Input: part model. Units: mm. Frame: model coordinates. A direction names the side the tool comes from. Give positions to 0.01 mm unless a question says otherwise; leave off trailing zeros. Order: outer loops, then holes, each group sorted by start corner. A loop starts at its lowest first (then second) coordinate and runs counter-clockwise, first axis right, second up. Notation, with made-up numbers: (44, 73) - (73, 73) arc R21 cw to (73, 90) - close; hole circle Ø3 at (29.25, -0.75). An arc over 180 degrees is marked (long way). Use a Markdown table: item, result.
from build123d import *

# Parameters (mm, degrees)
SKETCH1_W           = 22.9
SKETCH1_H           = 12.4968
BOSS_EXTRUDE1_DEPTH = 5.08
SKETCH2_W           = 22.9
SKETCH2_H           = 2.286
BOSS_EXTRUDE2_DEPTH = 1.016
SKETCH3_W           = 1.016
SKETCH3_H           = 1.016
CUT_EXTRUDE1_DEPTH  = 27.577930887
SKETCH4_W           = 20.2184
SKETCH4_H           = 2.4638
BOSS_EXTRUDE3_DEPTH = 6.8072
SKETCH5_W           = 7.62
SKETCH5_H           = 8.128
BOSS_EXTRUDE4_DEPTH = 2.8702
BOSS_EXTRUDE6_DEPTH = 1.778


with BuildPart() as part:
    # Sketch1 → Boss-Extrude1 (new body)
    with BuildSketch(Plane(origin=(0, 0, 0), x_dir=(1, 0, 0), z_dir=(0, 1, 0))):
        with Locations((11.45, 6.2484)):
            Rectangle(SKETCH1_W, SKETCH1_H)
    extrude(amount=BOSS_EXTRUDE1_DEPTH)

    # Sketch2 → Boss-Extrude2 (add)
    with BuildSketch(Plane.XY):
        with Locations((11.45, 2.449418531)):
            Rectangle(SKETCH2_W, SKETCH2_H)
    extrude(amount=BOSS_EXTRUDE2_DEPTH)

    # Sketch3 → Cut-Extrude1 (cut, through all)
    with BuildSketch(Plane(origin=(0, 5.08, 0), x_dir=(1, 0, 0), z_dir=(0, 1, 0))):
        with Locations((2.56, -0.508)):
            Rectangle(SKETCH3_W, SKETCH3_H)
        with Locations((5.1, -0.508)):
            Rectangle(SKETCH3_W, SKETCH3_H)
        with Locations((7.64, -0.508)):
            Rectangle(SKETCH3_W, SKETCH3_H)
        with Locations((10.18, -0.508)):
            Rectangle(SKETCH3_W, SKETCH3_H)
        with Locations((12.72, -0.508)):
            Rectangle(SKETCH3_W, SKETCH3_H)
        with Locations((15.26, -0.508)):
            Rectangle(SKETCH3_W, SKETCH3_H)
        with Locations((17.8, -0.508)):
            Rectangle(SKETCH3_W, SKETCH3_H)
        with Locations((20.34, -0.508)):
            Rectangle(SKETCH3_W, SKETCH3_H)
    extrude(amount=-CUT_EXTRUDE1_DEPTH, mode=Mode.SUBTRACT)

    # Sketch4 → Boss-Extrude3 (add)
    with BuildSketch(Plane(origin=(0, 0, -12.4968), x_dir=(-1, 0, 0), z_dir=(0, 0, -1))):
        with Locations((-11.45, 2.54)):
            Rectangle(SKETCH4_W, SKETCH4_H)
    extrude(amount=BOSS_EXTRUDE3_DEPTH)

    # Sketch5 → Boss-Extrude4 (add)
    with BuildSketch(Plane(origin=(0, 3.7719, 0), x_dir=(1, 0, 0), z_dir=(0, 1, 0))):
        with Locations((11.45, 12.6746)):
            Rectangle(SKETCH5_W, SKETCH5_H)
    extrude(amount=BOSS_EXTRUDE4_DEPTH)

    # Sketch6 → Boss-Extrude6 (add)
    # profile 1 of 4: a face of its own
    with BuildSketch(Plane(origin=(0, 3.7719, 0), x_dir=(1, 0, 0), z_dir=(0, 1, 0))):
        with BuildLine():
            add(Edge.make_bspline(
                [(12.764837987, 19.304), (12.764837987, 19.513213272), (12.713813556, 19.940397022), (12.430473546, 20.689983513), (11.84369856, 21.434451274), (10.99868157, 22.128872758), (10.114149769, 22.755114216), (9.290977221, 23.379772734), (8.634141686, 24.039902479), (8.28695824, 24.637071385), (8.136269303, 25.170420647), (8.107573693, 25.497240703), (8.107573693, 25.654)],
                knots=[0, 0, 0, 0, 0.0625, 0.125, 0.25, 0.375, 0.5, 0.625, 0.75, 0.875, 0.9375, 1, 1, 1, 1], degree=3))
            Line((8.107573693, 25.654), (8.107573693, 28.829))
            Line((8.107573693, 28.829), (5.821803018, 28.829))
            Line((5.821803018, 28.829), (5.821803018, 25.672693301))
            add(Edge.make_bspline(
                [(1.842837987, 19.304), (1.842837987, 22.316040756), (5.821803018, 22.055802608), (5.821803018, 25.672693301)],
                knots=[0, 0, 0, 0, 1, 1, 1, 1], degree=3))
            Line((1.842837987, 19.304), (2.604837987, 19.304))
            add(Edge.make_bspline(
                [(2.604837987, 19.304), (2.604837987, 19.436184229), (2.628829628, 19.717403115), (2.748821923, 20.134038551), (3.017012948, 20.581214899), (3.561863063, 21.101594101), (4.28319589, 21.642805815), (5.083141911, 22.269605528), (5.750459382, 22.975833182), (6.10677757, 23.58043805), (6.230115453, 23.859247989), (6.250774433, 23.908581669)],
                knots=[0, 0, 0, 0, 0.0625, 0.125, 0.25, 0.375, 0.5, 0.625, 0.75, 0.824094442, 0.839719442, 0.839719442, 0.839719442, 0.839719442], degree=3))
            add(Edge.make_bspline(
                [(6.250774433, 23.908581669), (6.271433413, 23.95791535), (6.316227133, 24.071064885), (6.41779978, 24.365489751), (6.480855857, 24.623522586), (6.514810758, 24.824299603)],
                knots=[0.839719442, 0.839719442, 0.839719442, 0.839719442, 0.855344442, 0.875, 0.928476516, 0.928476516, 0.928476516, 0.928476516], degree=3))
            add(Edge.make_bspline(
                [(6.300749052, 23.880300217), (6.391194329, 24.164866019), (6.464932294, 24.476628676), (6.514810758, 24.824299603)],
                knots=[0.790040378, 0.790040378, 0.790040378, 0.790040378, 0.909912617, 0.909912617, 0.909912617, 0.909912617], degree=3))
            add(Edge.make_bspline(
                [(4.382837987, 19.304), (4.382837987, 21.310686016), (5.704652562, 22.004816166), (6.300749052, 23.880300217)],
                knots=[0, 0, 0, 0, 0.790040378, 0.790040378, 0.790040378, 0.790040378], degree=3))
            Line((4.382837987, 19.304), (5.144837987, 19.304))
            add(Edge.make_bspline(
                [(5.144837987, 19.304), (5.144837987, 19.427793819), (5.158559892, 19.685949652), (5.231289869, 20.113666624), (5.394061657, 20.587818607), (5.695490865, 21.140525626), (6.088197228, 21.743923542), (6.524741922, 22.447977177), (6.93514926, 23.302596179), (7.174536626, 24.122966736), (7.269542471, 24.705079276), (7.293215165, 24.899470513), (7.299029307, 24.951977964)],
                knots=[0, 0, 0, 0, 0.0625, 0.125, 0.25, 0.375, 0.5, 0.625, 0.75, 0.875, 0.918103341, 0.933728341, 0.933728341, 0.933728341, 0.933728341], degree=3))
            add(Edge.make_bspline(
                [(7.299029307, 24.951977964), (7.304843448, 25.004485416), (7.327450173, 25.230534496), (7.341165481, 25.474360975), (7.345573693, 25.654)],
                knots=[0.933728341, 0.933728341, 0.933728341, 0.933728341, 0.949353341, 1, 1, 1, 1], degree=3))
            add(Edge.make_bspline(
                [(7.417250324, 24.951977964), (7.370695979, 25.171529954), (7.345573693, 25.404885005), (7.345573693, 25.654)],
                knots=[0.926554678, 0.926554678, 0.926554678, 0.926554678, 1, 1, 1, 1], degree=3))
            add(Edge.make_bspline(
                [(12.002837987, 19.304), (12.002837987, 21.609223862), (8.004559962, 22.182204254), (7.417250324, 24.951977964)],
                knots=[0, 0, 0, 0, 0.926554678, 0.926554678, 0.926554678, 0.926554678], degree=3))
            Line((12.002837987, 19.304), (12.764837987, 19.304))
        make_face()
        with BuildLine():
            add(Edge.make_bspline(
                [(6.514810758, 24.824299603), (6.520540217, 24.858178177), (6.563211161, 25.129441995), (6.583803018, 25.423501077), (6.583803018, 25.672693301)],
                knots=[0.928476516, 0.928476516, 0.928476516, 0.928476516, 0.9375, 1, 1, 1, 1], degree=3))
            add(Edge.make_bspline(
                [(6.514810758, 24.824299603), (6.552295837, 25.08558415), (6.576305195, 25.367149502), (6.583803018, 25.672693301)],
                knots=[0.909912617, 0.909912617, 0.909912617, 0.909912617, 1, 1, 1, 1], degree=3))
        make_face(mode=Mode.SUBTRACT)
    # profile 2 of 4: a face of its own
    with BuildSketch(Plane(origin=(0, 3.7719, 0), x_dir=(1, 0, 0), z_dir=(0, 1, 0))):
        with BuildLine():
            Line((7.299029307, 24.951977964), (7.417250324, 24.951977964))
            add(Edge.make_bspline(
                [(7.417250324, 24.951977964), (7.370695979, 25.171529954), (7.345573693, 25.404885005), (7.345573693, 25.654)],
                knots=[0.926554678, 0.926554678, 0.926554678, 0.926554678, 1, 1, 1, 1], degree=3))
            add(Edge.make_bspline(
                [(7.299029307, 24.951977964), (7.304843448, 25.004485416), (7.327450173, 25.230534496), (7.341165481, 25.474360975), (7.345573693, 25.654)],
                knots=[0.933728341, 0.933728341, 0.933728341, 0.933728341, 0.949353341, 1, 1, 1, 1], degree=3))
        make_face()
    # profile 3 of 4: a face of its own
    with BuildSketch(Plane(origin=(0, 3.7719, 0), x_dir=(1, 0, 0), z_dir=(0, 1, 0))):
        with BuildLine():
            Line((6.250774433, 23.908581669), (6.300749052, 23.880300217))
            add(Edge.make_bspline(
                [(6.300749052, 23.880300217), (6.391194329, 24.164866019), (6.464932294, 24.476628676), (6.514810758, 24.824299603)],
                knots=[0.790040378, 0.790040378, 0.790040378, 0.790040378, 0.909912617, 0.909912617, 0.909912617, 0.909912617], degree=3))
            add(Edge.make_bspline(
                [(6.250774433, 23.908581669), (6.271433413, 23.95791535), (6.316227133, 24.071064885), (6.41779978, 24.365489751), (6.480855857, 24.623522586), (6.514810758, 24.824299603)],
                knots=[0.839719442, 0.839719442, 0.839719442, 0.839719442, 0.855344442, 0.875, 0.928476516, 0.928476516, 0.928476516, 0.928476516], degree=3))
        make_face()
    # profile 4 of 4: a face of its own
    with BuildSketch(Plane(origin=(0, 3.7719, 0), x_dir=(1, 0, 0), z_dir=(0, 1, 0))):
        with BuildLine():
            add(Edge.make_bspline(
                [(6.514810758, 24.824299603), (6.552295837, 25.08558415), (6.576305195, 25.367149502), (6.583803018, 25.672693301)],
                knots=[0.909912617, 0.909912617, 0.909912617, 0.909912617, 1, 1, 1, 1], degree=3))
            add(Edge.make_bspline(
                [(6.514810758, 24.824299603), (6.520540217, 24.858178177), (6.563211161, 25.129441995), (6.583803018, 25.423501077), (6.583803018, 25.672693301)],
                knots=[0.928476516, 0.928476516, 0.928476516, 0.928476516, 0.9375, 1, 1, 1, 1], degree=3))
        make_face()
    extrude(amount=-BOSS_EXTRUDE6_DEPTH)


solid = part.part
1. Set-up query: faces 5 (the face through (3.8, 3.592, 0.5)), 6 (the face through (21.559, 3, -16)), 7 (the face through (5.608, 2.5, 0.5)), 8 (the face through (14, 1.306, 0.5)). Return all of +Z, -Z, +X, -X, +Y, -Y with unobstructed straight access to the full face (end or side cutting, diameter ignored); none if empty.
Response:
| item | result |
|---|---|
| face 5 | +Z, +X, -X, +Y |
| face 6 | -Z, +X, +Y, -Y |
| face 7 | +Z, +Y, -Y |
| face 8 | +Z, +X, -X, -Y |
2. Material intervals for line 1 along Y through (x, z) = (17.25, -13.5); line 2 along Z through (x, y) = (7, 4); line 3 along X through (y, z) = (3.5, -23.25), sorted ascending.
Response:
| item | result |
|---|---|
| line 1 | y = 1.31 to 3.77 |
| line 2 | z = -12.5 to 0 |
| line 3 | x = 4.94 to 5.9, 6.06 to 6.89, 8.36 to 9.48 |
3. Section query B-B (x = 14). Return loops of the section in (y, z), then the cut area to 3 significant figures.
Response:
| item | result |
|---|---|
| outline | (0, -12.5) - (1.31, -12.5) - (1.31, -19.3) - (3.77, -19.3) - (3.77, -16.74) - (6.64, -16.74) - (6.64, -8.61) - (5.08, -8.61) - (5.08, 0) - (3.59, 0) - (3.59, 1.02) - (1.31, 1.02) - (1.31, 0) - (0, 0) - close |
| area | 101 mm^2 |
4. Mould query, pull axis X, two halves, no side actions, for faces 1 (the face through (11, 0, -6)), 2 (the face through (8.148, 2.5, 0.5)), 3 (the face through (11.6, 2.6, -19.304)), 4 (the face through (0, 3, -6)). Classes: pulls with the +X half, pulls with the -X half, needs draft (parallel to the pull), parting line crosses it, or undercut.
Response:
| item | result |
|---|---|
| face 1 | needs draft |
| face 2 | undercut |
| face 3 | undercut |
| face 4 | pulls with the -X half |
5. Pin query (flat end, axial travel): pin 1 (0.5 mm diameter, centred on x = 1, z = 0.5, fed in from -Y); pin 2 (1 mm diameter, centred on x = 7.5, y = 6, fed in from +Z); pin 3 (2 mm diameter, centred on y = 2.5, z = -26.5, fed in from +X); pin 4 (5 mm diameter, centred on x = 15, z = -22, fed in from +Y). Return the tip coordinate at first contact, or that it passes through.
Response:
| item | result |
|---|---|
| pin 1 | stops at y = 1.31 |
| pin 2 | stops at z = -8.61 |
| pin 3 | stops at x = 8.11 |
| pin 4 | passes through |
6. Section query C-C (y = 4.5). Return loops of the section in (x, z), then the cut area to 4 significant figures.
Response:
| item | result |
|---|---|
| outline | (0, -12.5) - (7.64, -12.5) - (7.64, -16.74) - (15.26, -16.74) - (15.26, -12.5) - (22.9, -12.5) - (22.9, 0) - (0, 0) - close |
| area | 318.5 mm^2 |
7. Section query D-D (y = 2.75). State how many separate pieces and enclosed holes the cut face has, then the cut area to 3 significant figures.
Response:
| item | result |
|---|---|
| separate pieces | 1 |
| enclosed holes | 2 |
| area | 464 mm^2 |
8. Section query A-A (z = -9). Return loops of the section in (x, y).
Response:
| item | result |
|---|---|
| outline | (0, 0) - (22.9, 0) - (22.9, 5.08) - (15.26, 5.08) - (15.26, 6.64) - (7.64, 6.64) - (7.64, 5.08) - (0, 5.08) - close |
